Verification items for the finished model (mm, model axes). Face numbers are marked on the shaded views. A direction names the side the tool comes from. Coordinates: 2 decimals unless noted, no trailing zeros. Write each loop counter-clockwise with the first axis right and the second up, starting at its lowest first coordinate (ties: lowest second). Pieces come first, ordered by that corner, then holes. Notation, with made-up numbers: (44, 65.5) -> (68, 65.5) arc R24 cw to (68, 100.5) -> close; hole circle Ø1 at (-17, 38.25). An arc over 180 degrees is marked (long way). Answer in a Markdown table with one row per item.
```python
from build123d import *

# Parameters (mm, degrees)
SKETCH1_W                = 7.35
SKETCH1_H                = 6
BOSS_EXTRUDE1_DEPTH      = 4
BOSS_EXTRUDE2_DEPTH      = 2.5
F_3_0_3_DIAMETER_HOLE1_D = 3
FILLET1_R                = 20


# Read off the part's stored shape, not the designer's step: Boss-Extrude1
with BuildPart() as part:
    # Sketch1 → Revolve1 (revolve)
    with BuildSketch(Plane.XZ, mode=Mode.PRIVATE) as revolve1_sk:
        with Locations((3.675, 1)):
            Rectangle(SKETCH1_W, SKETCH1_H)
    revolve(revolve1_sk.sketch.rotate(Axis((0, 0, 4), (0, 0, -1)), 180), axis=Axis((0, 0, 4), (0, 0, -1)))

    # Boss-Extrude1 outline → Boss-Extrude1 (add)
    with BuildSketch(Plane.XY):
        with BuildLine():
            ThreePointArc((3.75, 23.9), (0, 24.928607748), (-3.75, 23.9))
            Line((-3.75, 23.9), (-3.75, 6.321392252))
            ThreePointArc((-3.75, 6.321392252), (0, 7.35), (3.75, 6.321392252))
            Line((3.75, 6.321392252), (3.75, 23.9))
        make_face()
    extrude(amount=BOSS_EXTRUDE1_DEPTH)

    # Sketch3 → Boss-Extrude2 (add)
    with BuildSketch(Plane(origin=(0, 0, 0), x_dir=(-1, 0, 0), z_dir=(0, 0, -1))):
        with BuildLine():
            Line((3, 23.9), (3, 19.9))
            ThreePointArc((3, 19.9), (0, 16.9), (-3, 19.9))
            Line((-3, 19.9), (-3, 23.9))
            ThreePointArc((-3, 23.9), (0, 26.9), (3, 23.9))
        make_face()
    extrude(amount=BOSS_EXTRUDE2_DEPTH)

    # Ø3.0 (3) Diameter Hole1 (through all)
    with Locations(Plane(origin=(0, 0, -2.5), x_dir=(-1, 0, 0), z_dir=(0, 0, -1))):
        with Locations((0, 23.9), (0, 19.9)):
            Hole(F_3_0_3_DIAMETER_HOLE1_D / 2)

    # Sketch6 → CBORE for M2.5 Hex Head Machine Screw1 (revolve, cut)
    with BuildSketch(Plane(origin=(0, 0, -2), x_dir=(0, 1, 0), z_dir=(1, 0, 0))):
        Polygon((0, 0), (0, 6), (3, 6), (1.5, 4.5), (1.5, 3), (3, 3), (3, 0), align=None)
    revolve(axis=Axis((0, 0, -8.35), (0, 0, 1)), mode=Mode.SUBTRACT)

    # Fillet1
    fillet1_edges = [part.edges().sort_by_distance(p)[0] for p in [
        (-3.75, 6.321392252, 2),
        (3.75, 6.321392252, 2),
    ]]
    fillet(fillet1_edges, radius=FILLET1_R)


solid = part.part
```
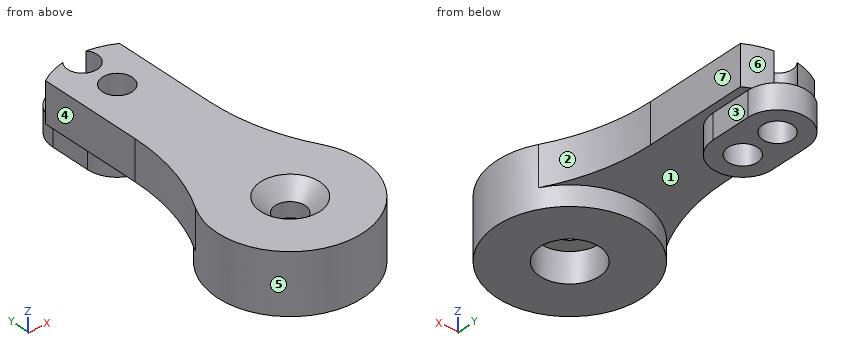
1. Go/stop test with flat-tipped pins: pin 1 (5 mm diameter, centred on x = -0.5, y = -0.5, fed in from -Z); pin 2 (2 mm diameter, centred on y = 19, z = 1.5, fed in from -X); pin 3 (2 mm diameter, centred on x = -1.5, y = 26, fed in from +Z). Record where each tip stops, or that it passes through.
Findings below:
| item | result |
|---|---|
| pin 1 | stops at z = -2 |
| pin 2 | stops at x = -3.75 |
| pin 3 | stops at z = 0 |
2. Sectioned sample at D-D, the plane x = 4.5. Record the cut outline in (y, z), and give its area (3 significant figures).
Findings below:
| item | result |
|---|---|
| outline | (-5.81, -2) -> (5.81, -2) -> (5.81, 0) -> (8.14, 0) -> (8.14, 4) -> (-5.81, 4) -> close |
| area | 79.0 mm² |
3. Sectioned sample at B-B, the plane y = 0. Record the cut outline in (x, z), and give its area (4 significant figures).
Findings below:
| item | result |
|---|---|
| outline | (-7.35, -2) -> (-3, -2) -> (-3, 1) -> (-1.5, 1) -> (-1.5, 2.5) -> (-3, 4) -> (-7.35, 4) -> close; (1.5, 1) -> (3, 1) -> (3, -2) -> (7.35, -2) -> (7.35, 4) -> (3, 4) -> (1.5, 2.5) -> close |
| area | 58.95 mm² |
4. Access from +Z, -Z, +X, -X, +Y, -Y to the whole of each face (thin tool, end or side, straight path). Record for the marked faces 4, 5, 6 and 7.
Findings below:
| item | result |
|---|---|
| face 4 | +Z, -Z, -X, +Y |
| face 5 | -Z |
| face 6 | +Z, +X, +Y |
| face 7 | +Z, -Z, +X, +Y |
5. Release check for a two-part mould opening along Y. For the marked faces 1, 2 and 3 record: released by +Y, released by -Y, zero draft, split by the parting line, or undercut.
Findings below:
| item | result |
|---|---|
| face 1 | undercut |
| face 2 | released by +Y |
| face 3 | zero draft |
6. Sectioned sample at A-A, the plane z = -0.75. Record the cut outline in (x, y), and give its area (3 significant figures).
Findings below:
| item | result |
|---|---|
| outline | circle Ø14.7 at (0, 0); (-3, 19.9) arc R3 ccw to (3, 19.9) -> (3, 23.9) arc R3 ccw to (-3, 23.9) -> close; hole circle Ø6 at (0, 0); hole circle Ø3 at (0, 19.9); hole circle Ø3 at (0, 23.9) |
| area | 180 mm² |
7. Sectioned sample at C-C, the plane z = 3. Record the cut outline in (x, y), and give its area (3 significant figures).
Findings below:
| item | result |
|---|---|
| outline | (-6.38, 3.64) arc R7.35 ccw (long way) to (6.38, 3.64) arc R20 cw to (3.75, 13.56) -> (3.75, 23.9) arc R7.35 ccw to (1.17, 24.83) arc R1.5 cw (long way) to (-1.17, 24.83) arc R7.35 ccw to (-3.75, 23.9) -> (-3.75, 13.56) arc R20 cw to start; hole circle Ø4 at (0, 0); hole circle Ø3 at (0, 19.9) |
| area | 284 mm² |
8. Material ranges on probe 1 along Y at (x, z) = (0, 2.25); probe 2 along Y at (x, z) = (1.75, -1.5); probe 3 along X at (y, z) = (0, 0.25), recorded low to high. Write a range as from..to.
Findings below:
| item | result |
|---|---|
| probe 1 | y = -7.35..-1.5, 1.5..18.4, 21.4..22.4 |
| probe 2 | y = -7.14..-2.44, 2.44..7.14, 17.46..26.34 |
| probe 3 | x = -7.35..-3, 3..7.35 |
